from build123d import *

# Parameters (mm, degrees)
F0_W     = 42
F0_H     = 42
F0_R     = 1.75
F0_R_2   = 11.25
F1_DEPTH = 4
F2_R     = 2
F2_W     = 42
F2_H     = 4
F3_DEPTH = 2.5
F4_SIZE  = 1.5


# Not quite as in the source:
# - a feature names something its author has since deleted; it is built from what else it names


with BuildPart() as f1:
    # F0 (on Top) → F1 (new body)
    with BuildSketch(Plane.XY):
        Rectangle(F0_W, F0_H)
        with Locations((-15.5, -15.5)):
            Circle(F0_R, mode=Mode.SUBTRACT)
        with Locations((15.5, -15.5)):
            Circle(F0_R, mode=Mode.SUBTRACT)
        with Locations((-15.5, 15.5)):
            Circle(F0_R, mode=Mode.SUBTRACT)
        Circle(F0_R_2, mode=Mode.SUBTRACT)
        with Locations((15.5, 15.5)):
            Circle(F0_R, mode=Mode.SUBTRACT)
    extrude(amount=-F1_DEPTH)

    # F2 (on face) → F3 (join)
    with BuildSketch(Plane.XZ.offset(21)):
        Polygon((50, -30), (50, 0), (21, 0), (21, -4), (-21, -4), (-21, 0), (-50, 0), (-50, -30), (-9, -30), (-9, -25), (9, -25), (9, -30), align=None)
        with Locations((-40, -24.5)):
            Circle(F2_R, mode=Mode.SUBTRACT)
        with Locations((40, -24.5)):
            Circle(F2_R, mode=Mode.SUBTRACT)
        with Locations((-30, -15)):
            Circle(F2_R, mode=Mode.SUBTRACT)
        with Locations((-40, -5.5)):
            Circle(F2_R, mode=Mode.SUBTRACT)
        with Locations((30, -15)):
            Circle(F2_R, mode=Mode.SUBTRACT)
        with Locations((40, -5.5)):
            Circle(F2_R, mode=Mode.SUBTRACT)
        with Locations((0, -2)):
            Rectangle(F2_W, F2_H)
    extrude(amount=F3_DEPTH)

    # F4
    f4_edges = [f1.edges().sort_by_distance(p)[0] for p in [
        (-21, 21, -2),
        (21, 21, -2),
        (-50, -22.25, 0),
        (-50, -22.25, -30),
        (50, -22.25, -30),
        (50, -22.25, 0),
        (-9, -22.25, -30),
        (9, -22.25, -30),
    ]]
    chamfer(f4_edges, length=F4_SIZE)


solid = f1.part
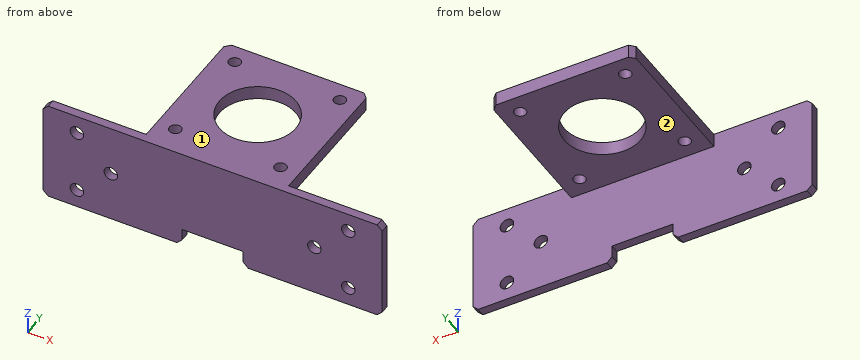
Read the model definition and answer for the solid it produces. Units are mm, in the model's axes. Face numbers are marked on the shaded views. A direction names the side the tool comes from. Round coordinates to 2 decimals unless told otherwise and drop trailing zeros. Write each loop counter-clockwise with the first axis right and the second up, starting at its lowest first coordinate (ties: lowest second). Pieces come first, ordered by that corner, then holes.
Q1. Find section B-B on y = -15.5. Determine the outline of the cut face in (x, z), and give its area (3 significant figures).
Values:
outline: (-21, -4) - (-17.25, -4) - (-17.25, 0) - (-21, 0) - close; (-13.75, -4) - (13.75, -4) - (13.75, 0) - (-13.75, 0) - close; (17.25, -4) - (21, -4) - (21, 0) - (17.25, 0) - close
area: 140 mm2
Q2. Straight lines are drawn through the part: line 1 (Z direction, x = -40, y = -21.8); line 2 (Y direction, x = -15.5, z = -2.85); line 3 (Y direction, x = 0, z = -2.1). For each, find the intervals that lie inside material, in ascending order.
Values:
line 1: z = -30 to -26.5, -22.5 to -7.5, -3.5 to 0
line 2: y = -23.5 to -17.25, -13.75 to 13.75, 17.25 to 21
line 3: y = -23.5 to -11.25, 11.25 to 21
Q3. Find section C-C on x = -30. Determine the outline of the cut face in (y, z), and give its area (3 significant figures).
Values:
outline: (-23.5, -30) - (-21, -30) - (-21, -17) - (-23.5, -17) - close; (-23.5, -13) - (-21, -13) - (-21, 0) - (-23.5, 0) - close
area: 65.0 mm2
Q4. A tool of negligible diameter and unlimited length cuts with its end or side. For the marked faces 1 and 2, from which of +Z, -Z, +X, -X, +Y, -Y can it reach the whole face along a straight path? Write none if from no direction.
Values:
face 1: +Z, +X, -X, +Y, -Y
face 2: -Z, +X, -X, +Y
Q5. Flat-ended cylindrical pins translate along their axes: P1, Ø2, axis at y = 8, z = -2.5, coming from the +X side; P2, Ø6.5, axis at x = -40, z = -24.5, coming from the +Y side; P3, Ø5, axis at x = -40, z = -5.5, coming from the -Y side; P4, Ø10, axis at x = -19, y = -8.5, coming from the -Z side. Find the tip coordinate at first contact, or state that the pin passes through.
Values:
P1: stops at x = 21
P2: stops at y = -21
P3: stops at y = -23.5
P4: stops at z = -4
Q6. Find section A-A on y = 0. Determine the outline of the cut face in (x, z), and give its area (3 significant figures).
Values:
outline: (-21, -4) - (-11.25, -4) - (-11.25, 0) - (-21, 0) - close; (11.25, -4) - (21, -4) - (21, 0) - (11.25, 0) - close
area: 78.0 mm2
Q7. Find section D-D on z = -5.5. Determine the outline of the cut face in (x, y).
Values:
outline: (-50, -23.5) - (-42, -23.5) - (-42, -21) - (-50, -21) - close; (-38, -23.5) - (38, -23.5) - (38, -21) - (-38, -21) - close; (42, -23.5) - (50, -23.5) - (50, -21) - (42, -21) - close
